Verification items for this drawing (mm, ordinates from the low corner). A direction names the side the tool comes from. Coordinates: 2 decimals unless noted, no trailing zeros. Order: outer loops, then holes, each group sorted by start corner. A loop starts at its lowest first (then second) coordinate and runs counter-clockwise, first axis right, second up. Notation, with made-up numbers: M 9.5,82 L 66.5,82 A26 cw 66.5,98 Z; hole C 63,-3.5 d10. An arc over 180 degrees is marked long. Use CSV: the item, a comma, the result in double quotes. Start each with the question number.
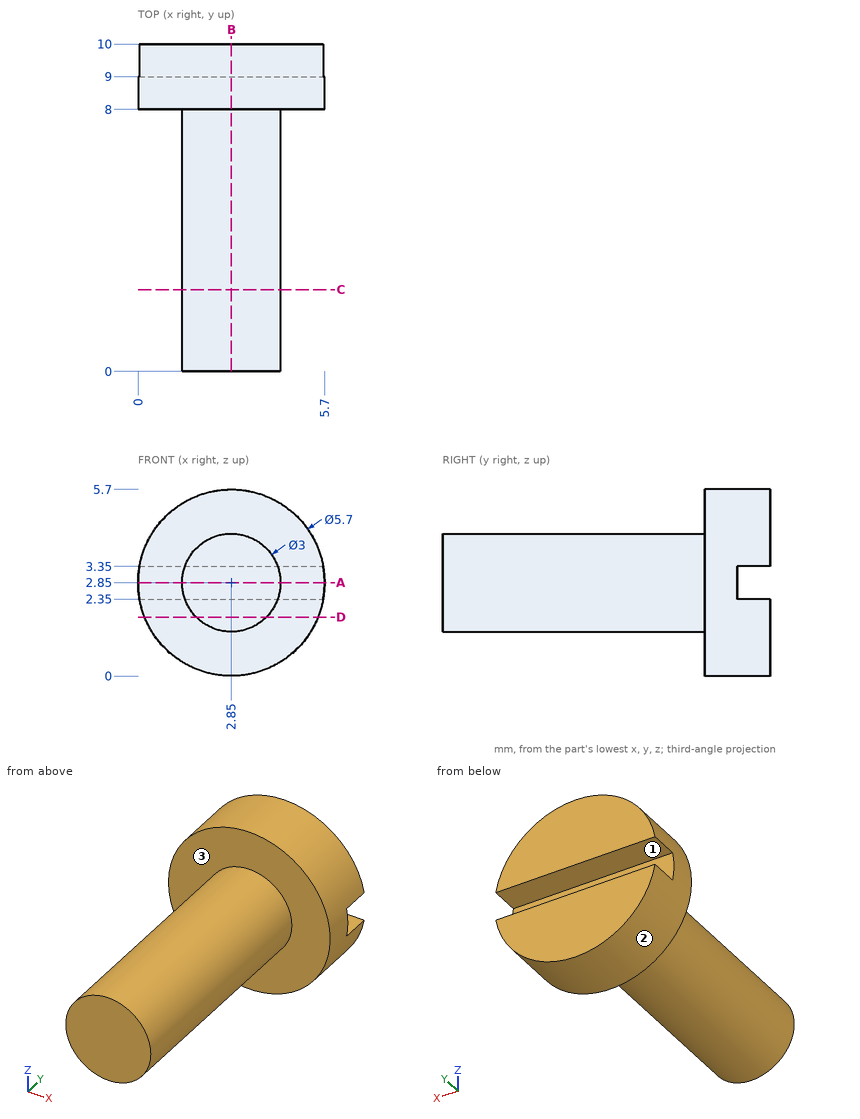
1) Section check A-A on z = 2.85. Record the boundary of the cut face in (x, y), then the cut area to 3 significant figures.
2) Gauge pin test, flat ends, axial feed: P1, Ø0.5, axis at x = 3, y = 9.5, coming from the +Z side; P2, Ø1.5, axis at y = 5, z = 3, coming from the +X side. Record the tip position at first contact, or that the pin passes through.
3) Set-up check for the marked faces 1, 2 and 3: record each of +Z, -Z, +X, -X, +Y, -Y from which the full face is reachable in a straight line by a thin tool's end or side.
4) Section check B-B on x = 2.85. Record the boundary of the cut face in (y, z).
5) Section check C-C on y = 2.5. Record the boundary of the cut face in (x, z), then the cut area to 3 significant figures.
6) Material ranges on line 1 along Y through (x, z) = (5.05, 4.6); line 2 along Z through (x, y) = (3.35, 9.25); line 3 along X through (y, z) = (2.25, 3.8), recorded low to high.
7) Section check D-D on z = 1.8. Record the boundary of the cut face in (x, y).
Results are:
1,outline,"M 0,8 L 1.35,8 L 1.35,0 L 4.35,0 L 4.35,8 L 5.7,8 L 5.7,9 L 0,9 Z"
1,area,"29.7 mm²"
2,P1,"stops at z = 5.7"
2,P2,"stops at x = 4.35"
3,face 1,"+X, -X, +Y"
3,face 2,"+Y, -Y"
3,face 3,"-Y"
4,outline,"M 0,1.35 L 8,1.35 L 8,0 L 10,0 L 10,2.35 L 9,2.35 L 9,3.35 L 10,3.35 L 10,5.7 L 8,5.7 L 8,4.35 L 0,4.35 Z"
5,outline,"C 2.85,2.85 d3"
5,area,"7.07 mm²"
6,line 1,"y = 8 to 10"
6,line 2,"z = 0.04 to 2.35, 3.35 to 5.66"
6,line 3,"x = 1.69 to 4.01"
7,outline,"M 0.2,8 L 1.78,8 L 1.78,0 L 3.92,0 L 3.92,8 L 5.5,8 L 5.5,10 L 0.2,10 Z"
